from build123d import *

# Parameters (mm, degrees)
F0_W     = 100
F0_H     = 37
F1_DEPTH = 5
F3_D     = 3.3
F5_D     = 8.5
F7_D     = 3.3
F7_DEPTH = 6
F7_TIP   = 0.9914200214


with BuildPart() as f1:
    # F0 (on Top) → F1 (new body)
    with BuildSketch(Plane.XY):
        Rectangle(F0_W, F0_H)
    extrude(amount=F1_DEPTH)

    # F3 (through all)
    with Locations(Plane.XY.offset(5)):
        with Locations((-36, 13), (-36, -13)):
            Hole(F3_D / 2)

    # F5 (through all)
    with Locations(Plane.XY.offset(5)):
        with Locations((-19, -10.5)):
            Hole(F5_D / 2)

    # F7
    with Locations(Plane.XY.offset(5)):
        with Locations((-6, 10), (-6, -10)):
            Hole(F7_D / 2, depth=F7_DEPTH)
            with Locations((0, 0, -(F7_DEPTH + F7_TIP / 2))):  # 118° drill point
                Cone(0, F7_D / 2, F7_TIP, mode=Mode.SUBTRACT)


solid = f1.part
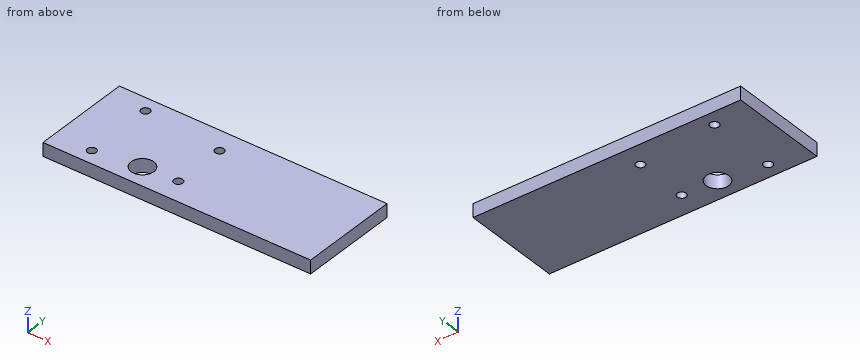
Verification items for the finished model (mm, model axes). Round coordinates to 2 decimals unless told otherwise and drop trailing zeros. Write each loop counter-clockwise with the first axis right and the second up, starting at its lowest first coordinate (ties: lowest second). Pieces come first, ordered by that corner, then holes.
(1) Material ranges on line 1 (Y direction, x = -36, z = 3.3); line 2 (Y direction, x = -6, z = 1.65); line 3 (X direction, y = -9, z = 2.5), recorded low to high.
Returned:
line 1: y = -18.5 to -14.65, -11.35 to 11.35, 14.65 to 18.5
line 2: y = -18.5 to -11.65, -8.35 to 8.35, 11.65 to 18.5
line 3: x = -50 to -22.98, -15.02 to -7.31, -4.69 to 50
(2) Section check C-C (z = 1.7). Enter the section's corners in (x, y).
Returned:
outline: (-50, -18.5) - (50, -18.5) - (50, 18.5) - (-50, 18.5) - close; hole circle Ø3.3 at (-36, -13); hole circle Ø3.3 at (-36, 13); hole circle Ø8.5 at (-19, -10.5); hole circle Ø3.3 at (-6, -10); hole circle Ø3.3 at (-6, 10)
(3) Section check A-A (x = -6). Enter the section's corners in (y, z), plus the area to 3 significant figures.
Returned:
outline: (-18.5, 0) - (-11.65, 0) - (-11.65, 5) - (-18.5, 5) - close; (-8.35, 0) - (8.35, 0) - (8.35, 5) - (-8.35, 5) - close; (11.65, 0) - (18.5, 0) - (18.5, 5) - (11.65, 5) - close
area: 152 mm2
(4) Section check D-D (x = -20). Enter the section's corners in (y, z), plus the area to 3 significant figures.
Returned:
outline: (-18.5, 0) - (-14.63, 0) - (-14.63, 5) - (-18.5, 5) - close; (-6.37, 0) - (18.5, 0) - (18.5, 5) - (-6.37, 5) - close
area: 144 mm2
(5) Section check B-B (y = 10). Enter the section's corners in (x, z).
Returned:
outline: (-50, 0) - (-7.65, 0) - (-7.65, 5) - (-50, 5) - close; (-4.35, 0) - (50, 0) - (50, 5) - (-4.35, 5) - close
(6) Depth check by flat-ended pin: pin 1 Ø4.5 at (x, y) = (-6, 10) entering from -Z. Enter the tip coordinate at first touch or a pass-through.
Returned:
pin 1: stops at z = 0
